Geometry check sheet. Reference: drawing and pictorial views, mm from the part's lowest x, y, z. A direction names the side the tool comes from. Round coordinates to 2 decimals unless told otherwise and drop trailing zeros. Write each loop counter-clockwise with the first axis right and the second up, starting at its lowest first coordinate (ties: lowest second). Pieces come first, ordered by that corner, then holes.
Item 1: Set-up check for the marked faces 1 and 2: record each of +Z, -Z, +X, -X, +Y, -Y from which the full face is reachable in a straight line by a thin tool's end or side.
Item 2: Material ranges on line 1 along Y through (x, z) = (15.56, 0.8); line 2 along Z through (x, y) = (21, 26); line 3 along X through (y, z) = (32.5, 1.5) (1 decimal), recorded low to high.
Item 3: Section check C-C, the plane x = 4.5. Record the cut outline in (y, z).
Item 4: Depth check by flat-ended pin: pin 1 (2 mm diameter, centred on x = 18.5, z = 4.5, fed in from +Y); pin 2 (2 mm diameter, centred on y = 8, z = 8.5, fed in from +X); pin 3 (4 mm diameter, centred on x = 15.56, y = 4.1, fed in from +Z). Enter the tip coordinate at first touch or a pass-through.
Item 5: Section check D-D, the plane z = 3. Record the cut outline in (x, y), plus the area to 3 significant figures.
Item 6: Section check B-B, the plane x = 15.56. Record the cut outline in (y, z).
Item 7: Section check A-A, the plane y = 33.4. Record the cut outline in (x, z).
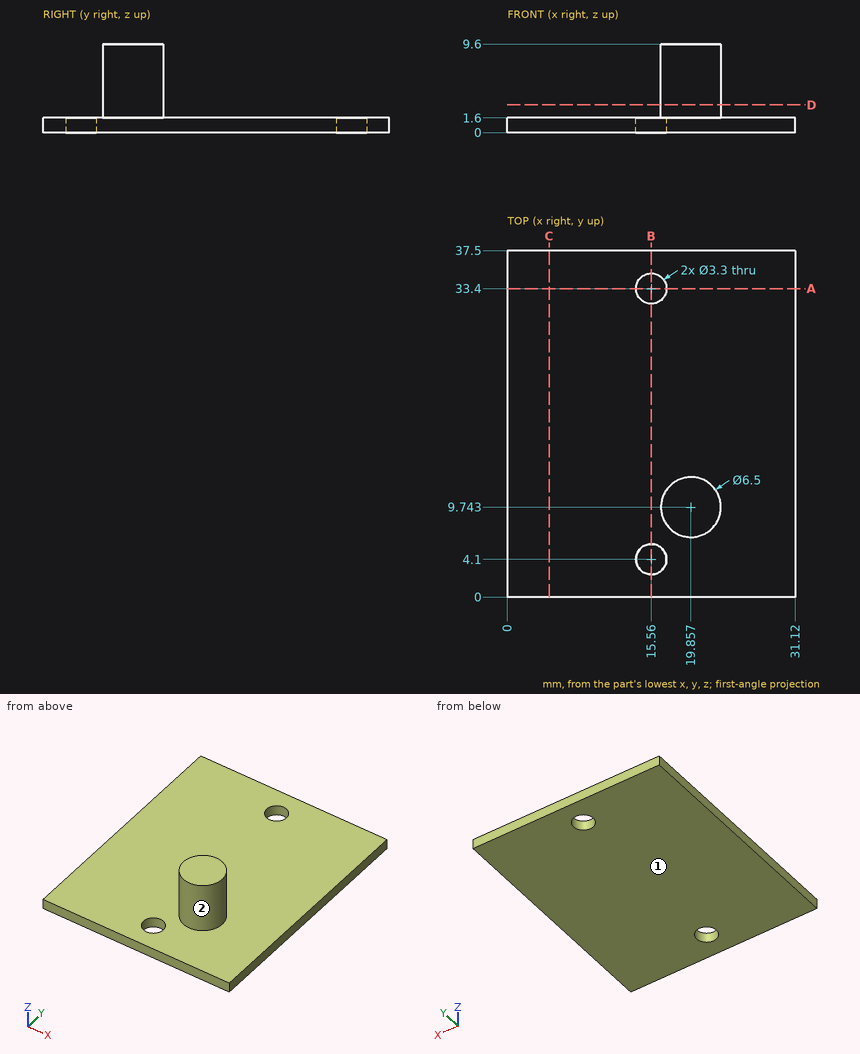
Values found:
1. face 1: -Z, +X, -X, +Y, -Y
1. face 2: +Z
2. line 1: y = 0 to 2.45, 5.75 to 31.75, 35.05 to 37.5
2. line 2: z = 0 to 1.6
2. line 3: x = 0 to 14.2, 16.9 to 31.1
3. outline: (0, 0) - (37.5, 0) - (37.5, 1.6) - (0, 1.6) - close
4. pin 1: stops at y = 12.97
4. pin 2: stops at x = 23.02
4. pin 3: stops at z = 1.6
5. outline: circle Ø6.5 at (19.86, 9.74)
5. area: 33.2 mm2
6. outline: (0, 0) - (2.45, 0) - (2.45, 1.6) - (0, 1.6) - close; (5.75, 0) - (31.75, 0) - (31.75, 1.6) - (5.75, 1.6) - close; (35.05, 0) - (37.5, 0) - (37.5, 1.6) - (35.05, 1.6) - close
7. outline: (0, 0) - (13.91, 0) - (13.91, 1.6) - (0, 1.6) - close; (17.21, 0) - (31.12, 0) - (31.12, 1.6) - (17.21, 1.6) - close
